```python
from build123d import *

# Parameters (mm, degrees)
CROQUIS1_W              = 100
CROQUIS1_H              = 60
CROQUIS1_R              = 6
CROQUIS1_R_2            = 1.5
SALIENTE_EXTRUIR1_DEPTH = 3
CROQUIS2_R              = 21.5
CROQUIS2_R_2            = 18.5
SALIENTE_EXTRUIR2_DEPTH = 20
CROQUIS4_W              = 100
CROQUIS4_H              = 60
CROQUIS4_R              = 21.5
SALIENTE_EXTRUIR3_DEPTH = 70
SALIENTE_EXTRUIR3_TAPER = 5


with BuildPart() as part:
    # Croquis1 → Saliente-Extruir1 (new body)
    with BuildSketch(Plane(origin=(0, 0, 0), x_dir=(1, 0, 0), z_dir=(0, 1, 0))):
        Rectangle(CROQUIS1_W, CROQUIS1_H)
        with Locations(Location((0, 7, 0), (0, 0, 270))):
            Circle(CROQUIS1_R, mode=Mode.SUBTRACT)
        with Locations(Location((15.5, 0, 0), (0, 0, 270))):
            Circle(CROQUIS1_R_2, mode=Mode.SUBTRACT)
        with Locations(Location((7.75, -13.423393759, 0), (0, 0, 270))):
            Circle(CROQUIS1_R_2, mode=Mode.SUBTRACT)
        with Locations(Location((-7.75, -13.423393759, 0), (0, 0, 270))):
            Circle(CROQUIS1_R_2, mode=Mode.SUBTRACT)
        with Locations(Location((-15.5, 0, 0), (0, 0, 270))):
            Circle(CROQUIS1_R_2, mode=Mode.SUBTRACT)
        with Locations(Location((-7.75, 13.423393759, 0), (0, 0, 270))):
            Circle(CROQUIS1_R_2, mode=Mode.SUBTRACT)
        with Locations(Location((7.75, 13.423393759, 0), (0, 0, 270))):
            Circle(CROQUIS1_R_2, mode=Mode.SUBTRACT)
    extrude(amount=SALIENTE_EXTRUIR1_DEPTH)

    # Croquis2 → Saliente-Extruir2 (add)
    with BuildSketch(Plane(origin=(0, 0, 0), x_dir=(1, 0, 0), z_dir=(0, 1, 0))):
        with Locations(Location((0, 0, 0), (0, 0, 270))):
            Circle(CROQUIS2_R)
        with Locations(Location((0, 0, 0), (0, 0, 270))):
            Circle(CROQUIS2_R_2, mode=Mode.SUBTRACT)
    extrude(amount=-SALIENTE_EXTRUIR2_DEPTH)

    # Croquis4 → Saliente-Extruir3 (add)
    with BuildSketch(Plane.XZ):
        Rectangle(CROQUIS4_W, CROQUIS4_H)
        with Locations(Location((0, 0, 0), (0, 0, 90))):
            Circle(CROQUIS4_R, mode=Mode.SUBTRACT)
    extrude(amount=SALIENTE_EXTRUIR3_DEPTH, taper=SALIENTE_EXTRUIR3_TAPER)


solid = part.part
```
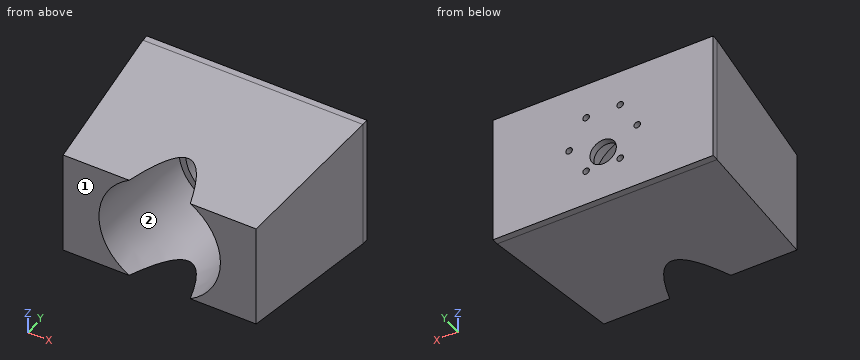
Build history of the part. All positions in model axes, mm. Face numbers are marked on the shaded views. Give positions to 0.01 mm unless a question says otherwise; leave off trailing zeros.
Item 1: Drill centre lines: line 1 (X direction, y = 2, z = 0); line 2 (X direction, y = -2, z = -13.5); line 3 (X direction, y = -5, z = 5). Where is each one in solid material? Low to high.
Answers follow:
line 1: x = -50 to -17, -14 to 14, 17 to 50
line 2: x = -49.83 to -16.96, -16.73 to -12.65, 12.65 to 16.73, 16.96 to 49.83
line 3: x = -49.56 to -21.36, -20.91 to -17.81, 17.81 to 20.91, 21.36 to 49.56
Item 2: Flat gauge pins, fed straight in: pin 1 (12 mm diameter, centred on x = 11, y = -16, fed in from -Z); pin 2 (12 mm diameter, centred on y = -7, z = -15.5, fed in from -X); pin 3 (2.5 mm diameter, centred on x = -7.75, z = 13.42, fed in from -Y); pin 4 (12 mm diameter, centred on y = -47.5, z = -21.5, fed in from +X). Where does each tip first touch, or does it go through?
Answers follow:
pin 1: stops at z = -29.13
pin 2: stops at x = -49.91
pin 3: passes through
pin 4: stops at x = 46.37
Item 3: Slice it at A-A, the plane x = -7.75. Give the number of separate pieces and of enclosed holes in the cut face, and give its area (3 significant figures).
Answers follow:
separate pieces: 3
enclosed holes: 0
area: 841 mm2
Item 4: Pull direction Z, two halves, no side cores. Call the marked faces 1 and 2: released by +Z, released by -Z, zero draft, split by the parting line, or undercut.
Answers follow:
face 1: zero draft
face 2: undercut
